Check sheet for the modelled part. Datum: model origin and axes. Units: mm. A direction names the side the tool comes from. Coordinates: 2 decimals unless noted, no trailing zeros. Loops run counter-clockwise (first coordinate to the right, second up) from the corner with the lowest first, then second, coordinate; pieces in that order, holes last. Notation, with made-up numbers: M 84.5,-3 L 122.5,-3 A11 cw 122.5,12 Z; hole C -13,60 d2. An arc over 180 degrees is marked long. Answer as CSV lines item,"result". Start each with the question number.
from build123d import *

# Parameters (mm, degrees)
F0_W        = 133.5890442133
F0_H        = 126.2129619718
F1_DEPTH    = 3.90208
F2_W        = 44.6898769587
F2_H        = 31.5666613169
F2_W_2      = 44.3351939321
F2_H_2      = 30.5026173592
F3_DEPTH    = 11.9221
F4_T        = 2.54
F4_T3_DEPTH = 49.4151939321
F4_T5_DEPTH = 35.5826173592
F4_T7_DEPTH = 49.7698769587
F4_T9_DEPTH = 36.6466613169


# Not quite as in the source:
# - a shell that OpenCascade refuses in one call is made with other operations: the cavity is built on its own and cut out


with BuildPart() as f1:
    # F0 (on Top) → F1 (new body)
    with BuildSketch(Plane.XY):
        with Locations((-0.6146728992, -2.3562498391)):
            Rectangle(F0_W, F0_H)
    extrude(amount=F1_DEPTH)

    # F2 (on face) → F3 (join)
    with BuildSketch(Plane.XY.offset(3.90208)):
        with Locations((0.623148866, 20.9897363093)):
            Rectangle(F2_W, F2_H)
        with Locations((0.8004903793, -28.4883454442)):
            Rectangle(F2_W_2, F2_H_2)
    extrude(amount=F3_DEPTH)

    # F4: shell of thickness 2.54, made by hand


with BuildPart() as f4_core1:
    # F4_t2: copy of F1
    add(f1.part)

    # the walls: a layer under each face that stays
    f4_faces = [f4_core1.faces().sort_by_distance(p)[0] for p in [
        (-0.6146728992, 60.7502311468, 1.95104),
        (66.1798492074, -2.3562498391, 1.95104),
        (-67.4091950059, -2.3562498391, 1.95104),
        (-0.6146728992, -2.3562498391, 0),
        (-0.6146728992, -2.3562498391, 3.90208),
        (-0.6146728992, -65.4627308249, 1.95104),
        (0.8004903793, -13.2370367646, 9.86313),
        (-21.3671065867, -28.4883454442, 9.86313),
        (0.8004903793, -43.7396541238, 9.86313),
        (22.9680873454, -28.4883454442, 9.86313),
        (0.623148866, 36.7730669677, 9.86313),
        (-21.7217896134, 20.9897363093, 9.86313),
        (0.623148866, 5.2064056508, 9.86313),
        (22.9680873454, 20.9897363093, 9.86313),
    ]]
    thicken(f4_faces, amount=-F4_T, mode=Mode.SUBTRACT)

    # F4_s4 → F4_t3 (cut)
    with BuildSketch(Plane.YZ.offset(-23.9071065867)):
        Polygon((-13.2116367646, 3.92748), (-13.2370367646, 1.36208), (-15.7770367646, 1.36208), (-15.7770367646, 3.90208), align=None)
        Polygon((-43.7650541238, 3.92748), (-43.7396541238, 1.36208), (-41.1996541238, 1.36208), (-41.1996541238, 3.90208), align=None)
    extrude(amount=F4_T3_DEPTH, mode=Mode.SUBTRACT)

    # F4_s6 → F4_t5 (cut)
    with BuildSketch(Plane.XZ.offset(10.6970367646)):
        Polygon((-21.3925065867, 3.92748), (-21.3671065867, 1.36208), (-18.8271065867, 1.36208), (-18.8271065867, 3.90208), align=None)
        Polygon((22.9934873454, 3.92748), (22.9680873454, 1.36208), (20.4280873454, 1.36208), (20.4280873454, 3.90208), align=None)
    extrude(amount=F4_T5_DEPTH, mode=Mode.SUBTRACT)

    # F4_s8 → F4_t7 (cut)
    with BuildSketch(Plane.YZ.offset(-24.2617896134)):
        Polygon((36.7984669677, 3.92748), (36.7730669677, 1.36208), (34.2330669677, 1.36208), (34.2330669677, 3.90208), align=None)
        Polygon((5.1810056508, 3.92748), (5.2064056508, 1.36208), (7.7464056508, 1.36208), (7.7464056508, 3.90208), align=None)
    extrude(amount=F4_T7_DEPTH, mode=Mode.SUBTRACT)

    # F4_s10 → F4_t9 (cut)
    with BuildSketch(Plane.XZ.offset(-39.3130669677)):
        Polygon((-21.7471896134, 3.92748), (-21.7217896134, 1.36208), (-19.1817896134, 1.36208), (-19.1817896134, 3.90208), align=None)
        Polygon((22.9934873454, 3.92748), (22.9680873454, 1.36208), (20.4280873454, 1.36208), (20.4280873454, 3.90208), align=None)
    extrude(amount=F4_T9_DEPTH, mode=Mode.SUBTRACT)


with BuildPart() as f1_1:
    add(f1.part)

    # what is left inside the walls is the cavity
    f4_cavity = [f4_core1.part.solids().sort_by_distance(p)[0] for p in [
        (0.80049, -32.725448, 2.5654),
        (0.623149, 16.575293, 2.5654),
    ]]
    add(f4_cavity, mode=Mode.SUBTRACT)


solid = f1_1.part
Item 1: Sectioned sample at D-D, the plane y = 31. Record the boundary of the cut face in (x, z).
Item 2: Sectioned sample at B-B, the plane y = -22.5. Record the boundary of the cut face in (x, z), and give its area (3 significant figures).
Item 3: Go/stop test with flat-tipped pins: pin 1 (4 mm diameter, centred on y = 26.5, z = 12, fed in from +X); pin 2 (2 mm diameter, centred on x = -24.5, z = 9.5, fed in from +Y); pin 3 (20.5 mm diameter, centred on x = -7.5, y = -29, fed in from +Z); pin 4 (3.5 mm diameter, centred on x = 7, z = 12.5, fed in from +Y). Record where each tip stops, or that it passes through.
Item 4: Material ranges on line 1 (Y direction, x = 7, z = 7); line 2 (X direction, y = 29.5, z = 13.25); line 3 (X direction, y = -36, z = 9.5), recorded low to high. Write a range as from..to.
Item 5: Release check for a two-part mould opening along X. For faces 4 (the face through (0, 34.233, 9)), 5 (the face through (1, -28, 2.54)), 6 (the face through (-67.409, -3, 2)), 7 (the face through (-2, 60.75, 2)) record: released by +X, released by -X, zero draft, split by the parting line, or undercut.
Item 6: Sectioned sample at C-C, the plane x = 27. Record the boundary of the cut face in (y, z).
Item 7: Sectioned sample at A-A, the plane z = 12.5. Record the boundary of the cut face in (x, y).
Item 8: Set-up check for faces 1 (the face through (-21.722, 21, 10)), 2 (the face through (1, -41.2, 9)), 3 (the face through (0, -43.74, 10)): record each of +Z, -Z, +X, -X, +Y, -Y from which the full face is reachable in a straight line by a thin tool's end or side.
Reply:
1,outline,"M -67.41,0 L 66.18,0 L 66.18,3.9 L 22.97,3.9 L 22.97,15.82 L 20.43,15.82 L 20.43,2.54 L -19.18,2.54 L -19.18,15.82 L -21.72,15.82 L -21.72,3.9 L -67.41,3.9 Z"
2,outline,"M -67.41,0 L 66.18,0 L 66.18,3.9 L 22.97,3.9 L 22.97,15.82 L 20.43,15.82 L 20.43,2.54 L -18.83,2.54 L -18.83,15.82 L -21.37,15.82 L -21.37,3.9 L -67.41,3.9 Z"
2,area,"528 mm²"
3,pin 1,"x = 22.97"
3,pin 2,"through"
3,pin 3,"z = 2.54"
3,pin 4,"y = 36.77"
4,line 1,"-43.74..-41.2, -15.78..-13.24, 5.21..7.75, 34.23..36.77"
4,line 2,"-21.72..-19.18, 20.43..22.97"
4,line 3,"-21.37..-18.83, 20.43..22.97"
5,face 4,"undercut"
5,face 5,"undercut"
5,face 6,"released by -X"
5,face 7,"zero draft"
6,outline,"M -65.46,0 L 60.75,0 L 60.75,3.9 L -65.46,3.9 Z"
7,outline,"M -21.72,5.21 L 22.97,5.21 L 22.97,36.77 L -21.72,36.77 Z; M -21.37,-43.74 L 22.97,-43.74 L 22.97,-13.24 L -21.37,-13.24 Z; hole M -19.18,7.75 L 20.43,7.75 L 20.43,34.23 L -19.18,34.23 Z; hole M -18.83,-41.2 L 20.43,-41.2 L 20.43,-15.78 L -18.83,-15.78 Z"
8,face 1,"+Z, -X, +Y, -Y"
8,face 2,"+Z"
8,face 3,"+Z, +X, -X, -Y"
